Work out the finished part from the listing and answer in its coordinate system (mm). A direction names the side the tool comes from. Give positions to 0.01 mm unless a question says otherwise; leave off trailing zeros. Order: outer loops, then holes, each group sorted by start corner. A loop starts at its lowest first (then second) coordinate and runs counter-clockwise, first axis right, second up. Notation, with made-up numbers: (8.25, -31) - (53.25, -31) arc R21 cw to (53.25, -1) - close; hole circle Ø6 at (-17, 72.25). An arc over 180 degrees is marked (long way). Put each result on its own line as item: value.
```python
from build123d import *

# Parameters (mm, degrees)
SKETCH1_R           = 1.6
SKETCH1_W           = 29
SKETCH1_H           = 32.7
BOSS_EXTRUDE1_DEPTH = 2
SKETCH2_W           = 29
SKETCH2_H           = 30.7
BOSS_EXTRUDE2_DEPTH = 2.8
SKETCH3_W           = 24.6
SKETCH3_H           = 16.6
CUT_EXTRUDE1_DEPTH  = 28.669522945
CHAMFER1_SIZE       = 1
CHAMFER2_SIZE       = 5
BOSS_EXTRUDE3_DEPTH = 19.8
FILLET1_R           = 1
FILLET2_R           = 2


with BuildPart() as part:
    # Sketch1 → Boss-Extrude1 (new body)
    # profile 1 of 3: a face of its own
    with BuildSketch(Plane.YZ):
        Polygon((14.5, -16.35), (21.8, 0), (14.5, 16.35), align=None)
        with Locations(Location((17.9, 0, 0), (0, 0, 270))):
            Circle(SKETCH1_R, mode=Mode.SUBTRACT)
    # profile 2 of 3: a face of its own
    with BuildSketch(Plane.YZ):
        Rectangle(SKETCH1_W, SKETCH1_H)
    # profile 3 of 3: a face of its own
    with BuildSketch(Plane.YZ):
        Polygon((-14.5, 16.35), (-21.8, 0), (-14.5, -16.35), align=None)
        with Locations(Location((-17.9, 0, 0), (0, 0, 270))):
            Circle(SKETCH1_R, mode=Mode.SUBTRACT)
    extrude(amount=BOSS_EXTRUDE1_DEPTH)

    # Sketch2 → Boss-Extrude2 (add)
    with BuildSketch(Plane.YZ.offset(2)):
        Rectangle(SKETCH2_W, SKETCH2_H)
    extrude(amount=BOSS_EXTRUDE2_DEPTH)

    # Sketch3 → Cut-Extrude1 (cut, through all)
    with BuildSketch(Plane.YZ.offset(4.8)):
        with Locations((0, 4.85)):
            Rectangle(SKETCH3_W, SKETCH3_H)
    extrude(amount=-CUT_EXTRUDE1_DEPTH, mode=Mode.SUBTRACT)

    # Chamfer1
    chamfer1_edges = [part.edges().sort_by_distance(p)[0] for p in [
        (2, -17.9, 1.6),
        (2, 17.9, 1.6),
    ]]
    chamfer(chamfer1_edges, length=CHAMFER1_SIZE)

    # Chamfer2
    chamfer2_edges = [part.edges().sort_by_distance(p)[0] for p in [
        (2.4, 12.3, 13.15),
        (2.4, -12.3, 13.15),
    ]]
    chamfer(chamfer2_edges, length=CHAMFER2_SIZE)

    # Sketch4 → Boss-Extrude3 (add)
    with BuildSketch(Plane(origin=(0, 0, 0), x_dir=(0, -1, 0), z_dir=(-1, 0, 0))):
        Polygon((-13.35, 10.4), (-13.35, -15.4), (13.35, -15.4), (13.35, 10.4), (8.35, 15.4), (-8.35, 15.4), align=None)
    extrude(amount=BOSS_EXTRUDE3_DEPTH)

    # Fillet1
    fillet1_edges = [part.edges().sort_by_distance(p)[0] for p in [
        (1, 14.5, -16.35),
        (1, -14.5, -16.35),
        (1, -21.8, 0),
        (1, -14.5, 16.35),
        (1, 14.5, 16.35),
        (1, 21.8, 0),
    ]]
    fillet(fillet1_edges, radius=FILLET1_R)

    # Fillet2
    fillet2_edges = [part.edges().sort_by_distance(p)[0] for p in [
        (3.4, -14.5, 15.35),
        (3.4, -14.5, -15.35),
        (3.4, 14.5, -15.35),
        (3.4, 14.5, 15.35),
    ]]
    fillet(fillet2_edges, radius=FILLET2_R)


solid = part.part
```
(1) A tool of negligible diameter and unlimited length cuts with its end or side. For faces 1 (the face through (-9.76, -10.88, 12.87)), 2 (the face through (-10, 0, -15.4)), 3 (the face through (2, -12.3, 2)), from which of +Z, -Z, +X, -X, +Y, -Y can it reach the whole face along a straight path? Write none if from no direction.
Geometry check:
face 1: +Z, -X, -Y
face 2: -Z, -X, +Y, -Y
face 3: +X
(2) Section B-B, the plane z = -9 is taken. Write down the section's boundary in (x, y), then the cut area to 3 significant figures.
Geometry check:
outline: (-19.8, -13.35) - (0, -13.35) - (0, -17.78) - (2, -17.78) - (2, -14.5) - (4.8, -14.5) - (4.8, 14.5) - (2, 14.5) - (2, 17.78) - (0, 17.78) - (0, 13.35) - (-19.8, 13.35) - close
area: 681 mm²
(3) Given pin 1 (1.4 mm diameter, centred on x = 1, z = 5, fed in from -Y); pin 2 (1.4 mm diameter, centred on x = 2.5, z = 1.5, fed in from +Y); pin 3 (10 mm diameter, centred on x = -8.5, y = 4.5, fed in from -Z); pin 4 (3 mm diameter, centred on y = 13.5, z = -0.5, fed in from -X), each flat-ended and moving along its own axis, determine where each tip first touches the part or whether it passes through.
Geometry check:
pin 1: stops at y = -19.88
pin 2: stops at y = 21.35
pin 3: stops at z = -15.4
pin 4: stops at x = -19.8
(4) Determine the mould class of faces 4 (the face through (2.434, 9.765, 10.685)), 5 (the face through (4.8, 0, -7)), 6 (the face through (3.42, 13.93, 14.75)) for opening direction Z: pulls with the +Z half, pulls with the -Z half, needs draft (parallel to the pull), parting line crosses it, or undercut.
Geometry check:
face 4: undercut
face 5: needs draft
face 6: pulls with the +Z half
(5) Section A-A, the plane y = -17.9 is taken. Write down the section's boundary in (x, z).
Geometry check:
outline: (0, -8.73) - (2, -8.73) - (2, -2.6) - (1, -1.6) - (0, -1.6) - close; (0, 1.6) - (1, 1.6) - (2, 2.6) - (2, 8.73) - (0, 8.73) - close
(6) Straight lines are drawn through the part: line 1 (Z direction, x = -2.5, y = 3); line 2 (Z direction, x = 1.25, y = -3); line 3 (Y direction, x = -11.25, z = -6). For each, find the intervals that lie inside material, in ascending order.
Geometry check:
line 1: z = -15.4 to 15.4
line 2: z = -16.35 to -3.45, 13.15 to 16.35
line 3: y = -13.35 to 13.35
(7) Section D-D, the plane x = -6.75 is taken. Write down the section's boundary in (y, z).
Geometry check:
outline: (-13.35, -15.4) - (13.35, -15.4) - (13.35, 10.4) - (8.35, 15.4) - (-8.35, 15.4) - (-13.35, 10.4) - close
(8) Section C-C, the plane y = 4.5 is taken. Write down the section's boundary in (x, z).
Geometry check:
outline: (-19.8, -15.4) - (0, -15.4) - (0, -16.35) - (2, -16.35) - (2, -15.35) - (4.8, -15.35) - (4.8, -3.45) - (0, -3.45) - (0, 13.15) - (4.8, 13.15) - (4.8, 15.35) - (2, 15.35) - (2, 16.35) - (0, 16.35) - (0, 15.4) - (-19.8, 15.4) - close
